Autodesk Inventor part; units mm, degrees
ref_plane "YZ Plane" through (0, 0, 0) normal (1, 0, 0) x (0, 1, 0)
ref_plane "XZ Plane" through (0, 0, 0) normal (0, 1, 0) x (-1, 0, 0)
ref_plane "XY Plane" through (0, 0, 0) normal (0, 0, 1) x (1, 0, 0)
sketch "스케치1" plane through (0, 0, 0) normal (0, 1, 0) x (-1, 0, 0)
  circle A0 centre (0, 0) radius 3.25
  dimension "d0" = 6.5
extrude "돌출1" add sketch "스케치1" along normal blind 50
sketch "스케치2" plane through (0, 0, 0) normal (0, 1, 0) x (-1, 0, 0)
  arc A0 (0, 5) -> (0, -5) centre (0, 0) ccw
  line L0 (0, 5) -> (0, -5)
  line L1 (0, -5.6) -> (0, 5.6)
  dimension "d3" = 10
revolve "회전1" add sketch "스케치2" angle 360 about axis through (0, 0, -10) along (0, 0, 1)
sketch "스케치3" plane through (0, 0, 0) normal (0, 0, 1) x (1, 0, 0)
  circle A0 centre (0, 0) radius 3.25
  dimension "d5" = 6.5
extrude "돌출2" add sketch "스케치3" along normal blind 50
sketch "스케치4" plane through (0, 0, 0) normal (1, 0, 0) x (0, 1, 0)
  circle A0 centre (0, 0) radius 3.25
  dimension "d8" = 6.5
extrude "돌출3" add sketch "스케치4" against normal blind 50
properties part number "arrows"
CAD build for the part. Positions are in the model's coordinates, mm. A direction names the side the tool comes from. Coordinates: 2 decimals unless noted, no trailing zeros. Loops run counter-clockwise (first coordinate to the right, second up) from the corner with the lowest first, then second, coordinate; pieces in that order, holes last. Notation, with made-up numbers: (18, 88.5) -> (44, 88.5) arc R36 ccw to (44, 126.5) -> close; hole circle Ø8 at (29, -24.75). An arc over 180 degrees is marked (long way). One line per item, written item: value.
1. Drill centre lines: line 1 (Z direction, x = -37, y = -1); line 2 (Y direction, x = -33.5, z = 1.5); line 3 (X direction, y = 0.5, z = 45.5). Where is each one in solid material? Low to high. Write a range as [from, to].
Answers:
line 1: z = [-3.09, 3.09]
line 2: y = [-2.88, 2.88]
line 3: x = [-3.21, 3.21]
2. Flat gauge pins, fed straight in: P1, Ø10, axis at x = -1.5, z = 15, coming from the -Y side; P2, Ø8, axis at y = 26, z = 5.5, coming from the +X side. Where does each tip first touch, or does it go through?
Answers:
P1: stops at y = -3.25
P2: stops at x = 2.88
3. Slice it at A-A on y = 0. Write the cut outline in (x, z), and give its area (3 significant figures).
Answers:
outline: (-50, -3.25) -> (-3.8, -3.25) arc R5 ccw (long way) to (3.25, 3.8) -> (3.25, 50) -> (-3.25, 50) -> (-3.25, 3.8) arc R5 ccw to (-3.8, 3.25) -> (-50, 3.25) -> close
area: 668 mm^2
4. Which spindle directions (+Z, -Z, +X, -X, +Y, -Y) get a long thin tool onto all of the face, cutting with end or side? Do faces 1 (the face through (0, 0, 50)), 2 (the face through (-26.576, -2.579, -1.978)), 3 (the face through (0, 50, 0)), 4 (the face through (-2.579, 1.978, 26.576)), 5 (the face through (2.579, 26.576, 1.978)). Say none if no direction does.
Answers:
face 1: +Z, +X, -X, +Y, -Y
face 2: -X
face 3: +Z, -Z, +X, -X, +Y
face 4: +Z
face 5: +Y
5. Slice it at C-C on x = -33. Write the cut outline in (y, z), and give its area (3 significant figures).
Answers:
outline: circle Ø6.5 at (0, 0)
area: 33.2 mm^2
